The model under review builds one solid part; all positions refer to its coordinate system, in mm. A direction names the side the tool comes from. Give positions to 0.01 mm unless a question says otherwise; leave off trailing zeros. Loops run counter-clockwise (first coordinate to the right, second up) from the corner with the lowest first, then second, coordinate; pieces in that order, holes last. Notation, with made-up numbers: M 73.5,86 L 129.5,86 A17 ccw 129.5,98 Z; hole C 53.25,68.25 d6. An arc over 180 degrees is marked long. One line per item, written item: value. Start each with the question number.
Q1. Mouldability with a two-part tool opening along Z and no side actions: class faces 4 (the face through (19.32, 8.42, 4.42)), 5 (the face through (19, 9, -3.175)), 6 (the face through (19, 1, 12.322)), 7 (the face through (38.1, 9, 3)) as released by +Z, released by -Z, zero draft, split by the parting line, or undercut.
Q2. We need section A-A on x = 34. Write out the cut boundary in (y, z) (1 decimal).
Q3. For faces 1 (the face through (19, 17, 12.322)), 2 (the face through (19, -0.833, 8)), 3 (the face through (19, 18.471, 8)), list the 3-axis set-ups (+Z, -Z, +X, -X, +Y, -Y) from which the entire face can be reached by the end or side of a thin tool; tool diameter is ignored.
Q4. We need section D-D on z = 7.5. Write out the cut boundary in (x, y), plus the area to 3 significant figures.
Q5. We need section B-B on z = 5.5. Write out the cut boundary in (x, y), plus the area to 3 significant figures.
Q6. We need section C-C on y = 20. Write out the cut boundary in (x, z) (3 decimals).
Q7. For pin 1 (5 mm diameter, centred on x = 12.5, y = 11, fed in from +Z); pin 2 (4 mm diameter, centred on x = 21.5, z = 9, fed in from +Y); pin 3 (4 mm diameter, centred on x = 34, z = 6, fed in from -Y), all flat-tipped, find the tip position at first contact; note any pin that passes through.
Q8. To check wall thickness, follow line 1 along Y through (x, z) = (6, 10.75); line 2 along Z through (x, y) = (15.5, -2) (3 decimals); line 3 along Y through (x, z) = (27, 5). State the ranges of each line that lie inside material, in increasing order. Write a range as from..to.
```python
from build123d import *

# Parameters (mm, degrees)
F0_W     = 19.304
F0_H     = 9.1468828812
F1_DEPTH = 38.1
F2_R     = 6.4726915954
F3_DEPTH = 38.1


with BuildPart() as f1:
    # F0 (on Right) → F1 (new body)
    with BuildSketch(Plane.YZ):
        with Locations((8.8194421337, 7.7484414406)):
            Rectangle(F0_W, F0_H)
        Polygon((-10.2305578663, -3.175), (27.8694421337, -3.175), (27.8694421337, 3.175), (18.4714421337, 3.175), (-0.8325578663, 3.175), (-10.2305578663, 3.175), align=None)
    extrude(amount=F1_DEPTH)

    # F2 (on face) → F3 (cut)
    with BuildSketch(Plane.YZ.offset(38.1)):
        with Locations((8.5852267221, 10.8897443861)):
            Circle(F2_R)
    extrude(amount=-F3_DEPTH, mode=Mode.SUBTRACT)


solid = f1.part
```
Solved:
1. face 4: undercut
1. face 5: released by -Z
1. face 6: released by +Z
1. face 7: zero draft
2. outline: M -10.2,-3.2 L 27.9,-3.2 L 27.9,3.2 L 18.5,3.2 L 18.5,12.3 L 14.9,12.3 A6.5 cw long 2.3,12.3 L -0.8,12.3 L -0.8,3.2 L -10.2,3.2 Z
3. face 1: +Z, +X, -X, +Y, -Y
3. face 2: +Z, +X, -X, -Y
3. face 3: +Z, +X, -X, +Y
4. outline: M 0,-0.83 L 38.1,-0.83 L 38.1,3.07 L 0,3.07 Z; M 0,14.1 L 38.1,14.1 L 38.1,18.47 L 0,18.47 Z
4. area: 315 mm2
5. outline: M 0,-0.83 L 38.1,-0.83 L 38.1,5 L 0,5 Z; M 0,12.17 L 38.1,12.17 L 38.1,18.47 L 0,18.47 Z
5. area: 462 mm2
6. outline: M 0,-3.175 L 38.1,-3.175 L 38.1,3.175 L 0,3.175 Z
7. pin 1: z = 6.68
7. pin 2: y = 18.47
7. pin 3: y = -0.83
8. line 1: -0.83..2.11, 15.06..18.47
8. line 2: -3.175..3.175
8. line 3: -0.83..5.9, 11.27..18.47
